from build123d import *

# Parameters (mm, degrees)
F0_W     = 50
F0_H     = 50
F0_R     = 1.5
F1_DEPTH = 1.6
F2_W     = 33.02
F2_H     = 17.78
F2_W_2   = 15.24
F2_H_2   = 12.7
F2_W_3   = 6.35
F2_H_3   = 23.1
F2_W_4   = 24.15
F2_W_5   = 7.62
F2_H_4   = 7.62
F2_W_6   = 15.86
F2_H_5   = 12.88
F3_DEPTH = 12
F5_W     = 43
F5_H     = 14.5
F6_DEPTH = 5
F7_R     = 0.5
F8_DEPTH = 6


with BuildPart() as f1:
    # F0 (on Top) → F1 (new body)
    with BuildSketch(Plane.XY):
        Rectangle(F0_W, F0_H)
        with Locations((-22.5, -22.5)):
            Circle(F0_R, mode=Mode.SUBTRACT)
        with Locations((22.5, -22.5)):
            Circle(F0_R, mode=Mode.SUBTRACT)
        with Locations((-22.5, 22.5)):
            Circle(F0_R, mode=Mode.SUBTRACT)
        with Locations((22.5, 22.5)):
            Circle(F0_R, mode=Mode.SUBTRACT)
    extrude(amount=F1_DEPTH)

    # F2 (on face) → F3 (join)
    with BuildSketch(Plane.XY.offset(1.6)):
        with Locations((5.95, -4.68)):
            Rectangle(F2_W, F2_H)
        with Locations((7.22, 12.3)):
            Rectangle(F2_W_2, F2_H_2)
        with Locations((-21.825, 6.87)):
            Rectangle(F2_W_3, F2_H_3)
        with Locations((-37.075, 6.87)):
            Rectangle(F2_W_4, F2_H_3)
        with Locations((-20.19, -11.03)):
            Rectangle(F2_W_5, F2_H_4)
        with Locations((-9.45, -31.44)):
            Rectangle(F2_W_6, F2_H_5)
        with Locations((-9.45, -21.19)):
            Rectangle(F2_W_6, F2_H_4)
    extrude(amount=F3_DEPTH)



with BuildPart() as f6:
    # F5 (on face) → F6 (new body)
    with BuildSketch(Plane(origin=(0, 11.7, -11.7), x_dir=(1, 0, 0), z_dir=(0, 0.707107, -0.707107))):
        with Locations((0, -29.25)):
            Rectangle(F5_W, F5_H)
    extrude(amount=-F6_DEPTH)


with BuildPart() as f1_1:
    add(f1.part)

    add(f6.part)  # F8 merges F6
    # F7 (on face) → F8 (join)
    with BuildSketch(Plane(origin=(0, 15.556349, 15.556349), x_dir=(1, 0, 0), z_dir=(0, -0.707107, -0.707107))):
        with Locations((15.5, -14.046299)):
            Circle(F7_R)
        with Locations((13.5, -14.046299)):
            Circle(F7_R)
        with Locations((11.5, -14.046299)):
            Circle(F7_R)
        with Locations((-15.5, -14.046299)):
            Circle(F7_R)
        with Locations((-13.5, -14.046299)):
            Circle(F7_R)
        with Locations((-11.5, -14.046299)):
            Circle(F7_R)
        with Locations((-9.5, -14.046299)):
            Circle(F7_R)
    extrude(amount=F8_DEPTH)


solid = f1_1.part
Can you work these out from the model? Positions are in its coordinate system, mm. A direction names the side the tool comes from. Give positions to 0.01 mm unless a question says otherwise; leave off trailing zeros. Loops run counter-clockwise (first coordinate to the right, second up) from the corner with the lowest first, then second, coordinate; pieces in that order, holes last. Notation, with made-up numbers: (69.25, -6) -> (77.25, -6) arc R14 cw to (77.25, -2) -> close; hole circle Ø1 at (87, 47.5). An arc over 180 degrees is marked (long way). Write item = value, one per line.
1) Suppose I cut it at C-C on x = 2. Write out the boundary of the cut face in (y, z), then the cut area to 3 significant figures.
Check result:
outline = (-25, 0) -> (25, 0) -> (25, 1.6) -> (18.65, 1.6) -> (18.65, 13.6) -> (5.95, 13.6) -> (5.95, 1.6) -> (4.21, 1.6) -> (4.21, 13.6) -> (-13.57, 13.6) -> (-13.57, 1.6) -> (-25, 1.6) -> close; (23.72, 7.39) -> (27.26, 3.86) -> (37.51, 14.11) -> (33.97, 17.64) -> close
area = 518 mm2
2) Suppose I cut it at A-A on x = -22.5. Write out the boundary of the cut face in (y, z).
Check result:
outline = (-25, 0) -> (-24, 0) -> (-24, 1.6) -> (-25, 1.6) -> close; (-21, 0) -> (21, 0) -> (21, 1.6) -> (18.42, 1.6) -> (18.42, 13.6) -> (-4.68, 13.6) -> (-4.68, 1.6) -> (-7.22, 1.6) -> (-7.22, 13.6) -> (-14.84, 13.6) -> (-14.84, 1.6) -> (-21, 1.6) -> close; (24, 0) -> (25, 0) -> (25, 1.6) -> (24, 1.6) -> close
3) Will these pins go through, and if not, where does the flat tip stop? pin 1 (2.5 mm diameter, centred on y = -11, z = 5, fed in from +X); pin 2 (1 mm diameter, centred on x = -28.5, z = 9.5, fed in from -Y); pin 3 (1 mm diameter, centred on x = -4.5, y = 26, fed in from +Z); pin 4 (2.5 mm diameter, centred on x = 22.5, y = 22.5, fed in from +Z).
Check result:
pin_1 = 22.46
pin_2 = -4.68
pin_3 = 10.17
pin_4 = through
4) Thinking about a two-plate mould opening in X: for faces 1 (the flat face through (6, 4.21, 8)), 2 (the flat face through (22.46, -5, 8)), 3 (the flat face through (-0.4, 12, 8)), which applies, released by +X, released by -X, zero draft, split by the parting line, or undercut?
Check result:
face_1 = zero draft
face_2 = released by +X
face_3 = undercut
5) Suppose I cut it at B-B on y = -22.5. Write out the boundary of the cut face in (x, z), then the cut area to 3 significant figures.
Check result:
outline = (-25, 0) -> (-24, 0) -> (-24, 1.6) -> (-25, 1.6) -> close; (-21, 0) -> (21, 0) -> (21, 1.6) -> (-1.52, 1.6) -> (-1.52, 13.6) -> (-17.38, 13.6) -> (-17.38, 1.6) -> (-21, 1.6) -> close; (24, 0) -> (25, 0) -> (25, 1.6) -> (24, 1.6) -> close
area = 261 mm2
6) For faces 4 (the flat face through (7, 5.95, 8)), 5 (the flat face through (-10, -31, 1.6)), 6 (the flat face through (7, 18.65, 8)), 7 (the flat face through (-1.52, -28, 8)), which set-ups out of +Z, -Z, +X, -X, +Y, -Y let a thin tool reach every point of the face, with its end or its side?
Check result:
face_4 = +Z, +X
face_5 = -Z, +X, -X, -Y
face_6 = +Z, +X, -X
face_7 = +Z, +X, -Y
7) Suppose I cut it at D-D on y = 15.5. Write out the boundary of the cut face in (x, z), then the cut area to 3 significant figures.
Check result:
outline = (-49.15, 1.6) -> (-25, 1.6) -> (-25, 0) -> (25, 0) -> (25, 1.6) -> (14.84, 1.6) -> (14.84, 13.6) -> (-0.4, 13.6) -> (-0.4, 1.6) -> (-18.65, 1.6) -> (-18.65, 13.6) -> (-49.15, 13.6) -> close
area = 629 mm2
8) I need wall thicknesses on L1, parallel to Y at x = 22.5, z = 0.6; L2, parallel to X at y = 13.5, z = 6; L3, parallel to X at y = 3.5, z = 3.5. Which ranges of each line are inside material? Lowest first, please. Write a range as from..to.
Check result:
L1 = -25..-24, -21..21, 24..25
L2 = -49.15..-18.65, -0.4..14.84
L3 = -49.15..-18.65, -10.56..22.46
